The drawing under review shows one solid part. Ordinate dimensions are in mm from its lowest x, y, z. A direction names the side the tool comes from. Round coordinates to 2 decimals unless told otherwise and drop trailing zeros. Write each loop counter-clockwise with the first axis right and the second up, starting at its lowest first coordinate (ties: lowest second). Pieces come first, ordered by that corner, then holes. Notation, with made-up numbers: (9.25, 12) -> (44.25, 12) arc R24 ccw to (44.25, 49) -> close; hole circle Ø11 at (59.5, -37.5). An arc over 180 degrees is marked (long way). Answer in a Markdown table with one row per item. Add a question column.
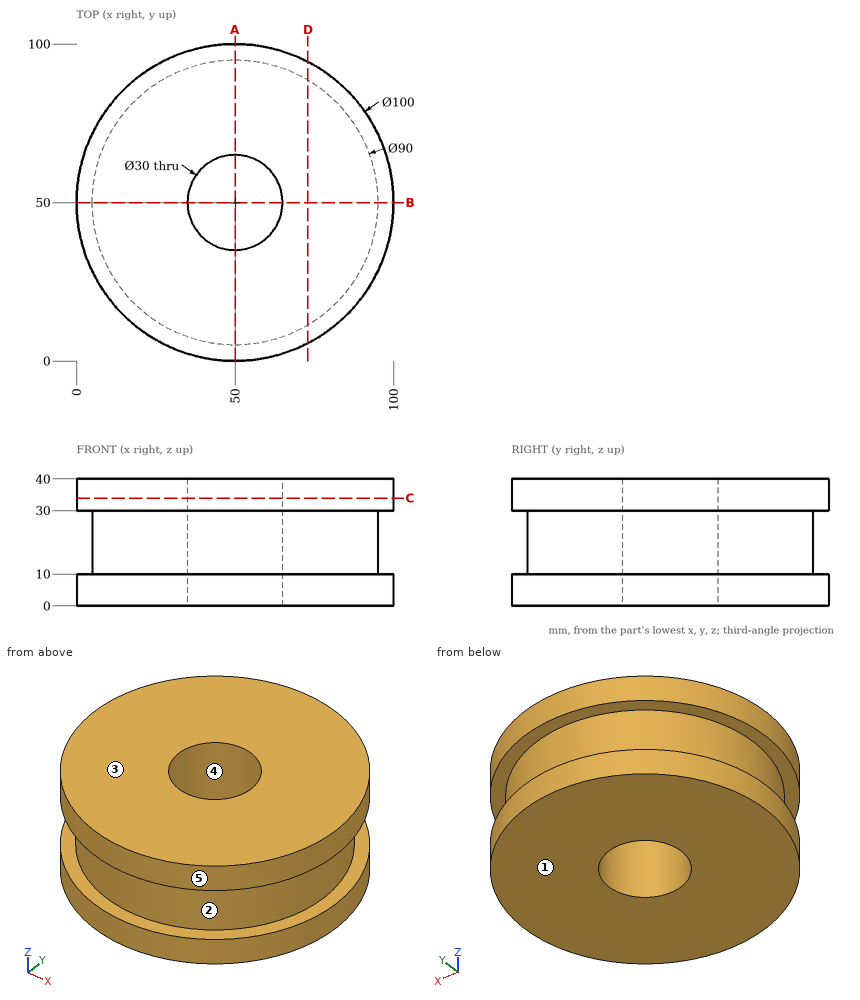
1. Add section A-A on x = 50. Write out the cut boundary in (y, z), plus the area to 3 significant figures.
2. Mouldability with a two-part tool opening along X and no side actions: class the marked faces 3, 4 and 5 as pulls with the +X half, pulls with the -X half, needs draft (parallel to the pull), parting line crosses it, or undercut.
3. Tool access review of the marked faces 1 and 2: name each direction out of +Z, -Z, +X, -X, +Y, -Y from which nothing blocks a thin tool from reaching the whole face with its end or side.
4. Add section C-C on z = 34. Write out the cut boundary in (x, y), plus the area to 3 significant figures.
5. Insertion check: pin 1 Ø8 at (y, z) = (59, 32) entering from -X; pin 2 Ø1.5 at (x, z) = (62, 16.5) entering from +Y; pin 3 Ø5 at (x, z) = (58, 29) entering from -Y; pin 4 Ø18 at (x, y) = (50, 50) entering from -Z. Each pin has a flat end and moves straight along its axis. Give the tip position at first contact, or say it passes through.
6. For L1, parallel to Y at x = 50, z = 8; L2, parallel to Z at x = 91.5, y = 26.5; L3, parallel to Y at x = 50, z = 18, list the stretches that pass through material, from the lowest coordinate up.
7. Add section D-D on x = 73. Write out the cut boundary in (y, z), plus the area to 3 significant figures.
Filled in:
| question | item | result |
|---|---|---|
| 1 | outline | (0, 0) -> (35, 0) -> (35, 40) -> (0, 40) -> (0, 30) -> (5, 30) -> (5, 10) -> (0, 10) -> close; (65, 0) -> (100, 0) -> (100, 10) -> (95, 10) -> (95, 30) -> (100, 30) -> (100, 40) -> (65, 40) -> close |
| 1 | area | 2,600 mm² |
| 2 | face 3 | needs draft |
| 2 | face 4 | undercut |
| 2 | face 5 | parting line crosses it |
| 3 | face 1 | -Z, +X, -X, +Y, -Y |
| 3 | face 2 | none |
| 4 | outline | circle Ø100 at (50, 50); hole circle Ø30 at (50, 50) |
| 4 | area | 7,150 mm² |
| 5 | pin 1 | x = 0.25 |
| 5 | pin 2 | y = 93.57 |
| 5 | pin 3 | y = 0.33 |
| 5 | pin 4 | through |
| 6 | L1 | 0 to 35, 65 to 100 |
| 6 | L2 | 0 to 10, 30 to 40 |
| 6 | L3 | 5 to 35, 65 to 95 |
| 7 | outline | (5.6, 0) -> (94.4, 0) -> (94.4, 10) -> (88.68, 10) -> (88.68, 30) -> (94.4, 30) -> (94.4, 40) -> (5.6, 40) -> (5.6, 30) -> (11.32, 30) -> (11.32, 10) -> (5.6, 10) -> close |
| 7 | area | 3,320 mm² |
